Input: part model. Units: mm. Frame: model coordinates. Face numbers are marked on the shaded views. A direction names the side the tool comes from. Give positions to 0.01 mm unless a question says otherwise; leave off trailing zeros. Loops run counter-clockwise (first coordinate to the right, second up) from the corner with the lowest first, then second, coordinate; pieces in that order, holes last. Notation, with made-up numbers: (-15.5, 85.5) - (27.5, 85.5) arc R15 cw to (27.5, 96.5) - close; hole circle Ø9 at (26, -28.75). An arc over 180 degrees is marked (long way). One line per item, written item: value.
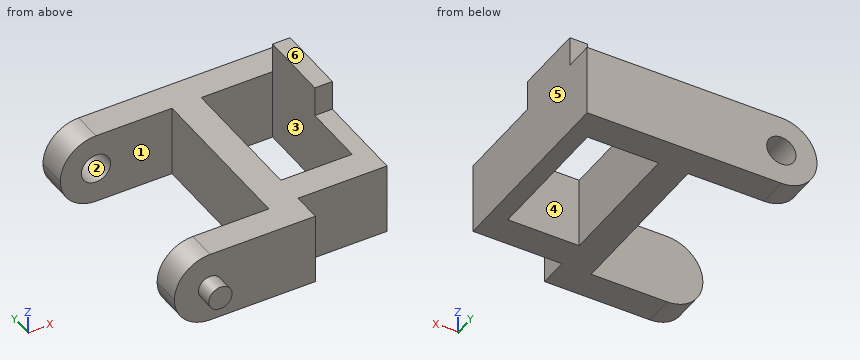
from build123d import *

# Parameters (mm, degrees)
BOSS_EXTRUDE1_DEPTH = 12.2
SKETCH4_R           = 2.5
CUT_EXTRUDE1_DEPTH  = 5
CUT_EXTRUDE2_START  = -38
CUT_EXTRUDE2_DEPTH  = 38
SKETCH6_R           = 2
BOSS_EXTRUDE2_DEPTH = 3
SKETCH7_W           = 12.2
SKETCH7_H           = 4.999065242
SKETCH7_H_2         = 5
BOSS_EXTRUDE3_DEPTH = 15.2
BOSS_EXTRUDE5_REACH = 57.477
SKETCH9_W           = 3
SKETCH9_H           = 12.2
SKETCH10_W          = 3
SKETCH10_H          = 12.2
BOSS_EXTRUDE6_DEPTH = 5.15


# Read off the part's stored shape, not the designer's step: Cut-Extrude2
with BuildPart() as part:
    # Sketch3 → Boss-Extrude1 (new body)
    with BuildSketch(Plane.XY):
        Polygon((-40.407881927, 21.413178882), (-21.307881927, 21.413178882), (-21.307881927, -6.586821118), (-40.407881927, -6.586821118), (-40.407881927, -11.586821118), (-16.307881927, -11.586821118), (-16.307881927, 26.413178882), (-40.407881927, 26.413178882), align=None)
    extrude(amount=BOSS_EXTRUDE1_DEPTH)

    # Sketch4 → Cut-Extrude1 (cut)
    with BuildSketch(Plane(origin=(0, 26.413178882, 0), x_dir=(1, 0, 0), z_dir=(0, 1, 0))):
        with Locations(Location((-34.307881927, -6.1, 0), (0, 0, 270))):
            Circle(SKETCH4_R)
    extrude(amount=-CUT_EXTRUDE1_DEPTH, mode=Mode.SUBTRACT)

    # Cut-Extrude2 outline → Cut-Extrude2 (cut)
    with BuildSketch(Plane(origin=(0, 26.413178882, 0), x_dir=(1, 0, 0), z_dir=(0, 1, 0)).offset(CUT_EXTRUDE2_START)):
        with BuildLine():
            Line((-40.407881927, -12.2), (-34.307881927, -12.2))
            ThreePointArc((-34.307881927, -12.2), (-38.621233292, -10.413351365), (-40.407881927, -6.1))
            Line((-40.407881927, -6.1), (-40.407881927, -12.2))
        make_face()
        with BuildLine():
            Line((-40.407881927, 0), (-40.407881927, -6.1))
            ThreePointArc((-40.407881927, -6.1), (-38.621233292, -1.786648635), (-34.307881927, 0))
            Line((-34.307881927, 0), (-40.407881927, 0))
        make_face()
    extrude(amount=CUT_EXTRUDE2_DEPTH, mode=Mode.SUBTRACT)

    # Sketch6 → Boss-Extrude2 (add)
    with BuildSketch(Plane.XZ.offset(11.586821118)):
        with Locations(Location((-34.307881927, 6.1, 0), (0, 0, 180))):
            Circle(SKETCH6_R)
    extrude(amount=BOSS_EXTRUDE2_DEPTH)

    # Sketch7 → Boss-Extrude3 (add)
    with BuildSketch(Plane(origin=(-16.307881927, 0, 0), x_dir=(0, 0, -1), z_dir=(1, 0, 0))):
        with Locations((-6.1, 23.913646261)):
            Rectangle(SKETCH7_W, SKETCH7_H)
        with Locations((-6.1, -4.086821118)):
            Rectangle(SKETCH7_W, SKETCH7_H_2)
    extrude(amount=BOSS_EXTRUDE3_DEPTH)

    # Sketch9 → Boss-Extrude5 (add, up to next)
    with BuildSketch(Plane.XZ.offset(-21.41411364), mode=Mode.PRIVATE) as boss_extrude5_sk1:
        with Locations((-2.607881927, 6.1)):
            Rectangle(SKETCH9_W, SKETCH9_H)
    boss_extrude5_tool1 = extrude(boss_extrude5_sk1.sketch, amount=BOSS_EXTRUDE5_REACH, mode=Mode.PRIVATE) - part.part
    add(boss_extrude5_tool1.solids().sort_by_distance((-2.607882, 21.414114, 6.1))[0])

    # Sketch10 → Boss-Extrude6 (add)
    with BuildSketch(Plane.XY.offset(12.2)):
        with Locations((-2.607881927, 15.31411364)):
            Rectangle(SKETCH10_W, SKETCH10_H)
    extrude(amount=BOSS_EXTRUDE6_DEPTH)


solid = part.part
Item 1: Material intervals for L1, parallel to X at y = 15.5, z = 11.5; L2, parallel to X at y = 24.6, z = 6.1; L3, parallel to Y at x = -29.5, z = 10, sorted ascending.
Verdict:
L1: x = -21.31 to -16.31, -4.11 to -1.11
L2: x = -40.41 to -36.81, -31.81 to -1.11
L3: y = -11.59 to -6.59, 21.41 to 26.41
Item 2: Section C-C, the plane z = 6.75. Output: boundary loops of the cut face in (x, y), and give its area (3 significant figures).
Verdict:
outline: (-40.37, -11.59) - (-36.2, -11.59) - (-36.2, -14.59) - (-32.42, -14.59) - (-32.42, -11.59) - (-16.31, -11.59) - (-16.31, -6.59) - (-1.11, -6.59) - (-1.11, 26.41) - (-31.89, 26.41) - (-31.89, 21.41) - (-21.31, 21.41) - (-21.31, -6.59) - (-40.37, -6.59) - close; (-40.37, 21.41) - (-36.72, 21.41) - (-36.72, 26.41) - (-40.37, 26.41) - close; hole (-16.31, -1.59) - (-4.11, -1.59) - (-4.11, 21.41) - (-16.31, 21.41) - close
area: 589 mm^2
Item 3: Section A-A, the plane x = -15.5. Output: boundary loops of the cut face in (y, z), and give its area (3 significant figures).
Verdict:
outline: (-6.59, 0) - (-1.59, 0) - (-1.59, 12.2) - (-6.59, 12.2) - close; (21.41, 0) - (26.41, 0) - (26.41, 12.2) - (21.41, 12.2) - close
area: 122 mm^2
Item 4: Access query for the marked faces 1, 2 and 3. Directions: +Z, -Z, +X, -X, +Y, -Y. A direction counts if a zero-diameter tool reaches every point of the face in a straight line with its end or side. Return the directions, or none.
Verdict:
face 1: +Z, -Z, -X
face 2: +Y
face 3: +Z, -Z
Item 5: Section B-B, the plane y = 13.5. Output: boundary loops of the cut face in (x, z), and give its area (3 significant figures).
Verdict:
outline: (-21.31, 0) - (-16.31, 0) - (-16.31, 12.2) - (-21.31, 12.2) - close; (-4.11, 0) - (-1.11, 0) - (-1.11, 17.35) - (-4.11, 17.35) - close
area: 113 mm^2
Item 6: Draft query along X for the marked faces 4, 5 and 6. Return one class per face: pulls with the +X half, pulls with the -X half, needs draft (parallel to the pull), parting line crosses it, or undercut.
Verdict:
face 4: undercut
face 5: pulls with the +X half
face 6: needs draft
Item 7: Section D-D, the plane y = 23. Output: boundary loops of the cut face in (x, z).
Verdict:
outline: (-34.31, 0) - (-1.11, 0) - (-1.11, 12.2) - (-34.31, 12.2) arc R6.1 ccw to start; hole circle Ø5 at (-34.31, 6.1)
Item 8: Pin query (flat end, axial travel): P1, Ø2.5, axis at x = -2, z = 14.5, coming from the -Y side; P2, Ø1, axis at y = 10.5, z = 10, coming from the -X side; P3, Ø1.5, axis at x = -8.5, z = 9.5, coming from the -Y side. Return the tip coordinate at first contact, or that it passes through.
Verdict:
P1: stops at y = 9.21
P2: stops at x = -21.31
P3: stops at y = -6.59
